```python
from build123d import *

# Parameters (mm, degrees)
SKETCH_1_R      = 2
SKETCH_1_R_2    = 9.5
EXTRUDE_2_DEPTH = 1.5


with BuildPart() as part:
    # 草图1 → 凸台-拉伸2 (new, symmetric)
    # profile 1 of 2: a face of its own
    with BuildSketch(Plane.XY):
        with BuildLine():
            Line((-30, 12.5), (-30, -22.5))
            Line((-30, -22.5), (30, -22.5))
            Line((30, -22.5), (30, 22.5))
            Line((30, 22.5), (-20, 22.5))
            Line((-20, 22.5), (-20, 14.5))
            ThreePointArc((-20, 14.5), (-18.585786438, 13.914213562), (-18, 12.5))
            ThreePointArc((-18, 12.5), (-20, 10.5), (-22, 12.5))
            Line((-22, 12.5), (-30, 12.5))
        make_face()
        with Locations((-20, -12.5)):
            Circle(SKETCH_1_R, mode=Mode.SUBTRACT)
        with Locations((20, -12.5)):
            Circle(SKETCH_1_R, mode=Mode.SUBTRACT)
        with Locations((0, 2.5)):
            Circle(SKETCH_1_R_2, mode=Mode.SUBTRACT)
        with Locations((20, 12.5)):
            Circle(SKETCH_1_R, mode=Mode.SUBTRACT)
    # profile 2 of 2: a face of its own
    with BuildSketch(Plane.XY):
        with BuildLine():
            Line((-30, 22.5), (-30, 12.5))
            Line((-30, 12.5), (-22, 12.5))
            ThreePointArc((-22, 12.5), (-21.414213562, 13.914213562), (-20, 14.5))
            Line((-20, 14.5), (-20, 22.5))
            Line((-20, 22.5), (-30, 22.5))
        make_face()
    extrude(amount=EXTRUDE_2_DEPTH, both=True)


solid = part.part
```
Geometry check sheet. Reference: the model listing, model coordinates, mm. Round coordinates to 2 decimals unless told otherwise and drop trailing zeros. Order: outer loops, then holes, each group sorted by start corner. A loop starts at its lowest first (then second) coordinate and runs counter-clockwise, first axis right, second up. Notation, with made-up numbers: (84, 14) - (114, 14) arc R13 cw to (114, 31) - close; hole circle Ø3 at (5, -30). An arc over 180 degrees is marked (long way). Use a Markdown table: item, result. Add a question column.
(1) Sectioned sample at C-C, the plane x = 20. Enter the section's corners in (y, z), and give its area (3 significant figures).
(2) Sectioned sample at B-B, the plane y = -12.5. Enter the section's corners in (x, z).
(3) Release check for a two-part mould opening along Y. For faces 1 (the cylindrical face through (19.74, 14.483, -0.021)), 2 (the flat face through (0, -22.5, 0)), 3 (the flat face through (-30, 0, 0)) record: pulls with the +Y half, pulls with the -Y half, needs draft (parallel to the pull), parting line crosses it, or undercut.
(4) Sectioned sample at A-A, the plane x = 0. Enter the section's corners in (y, z).
(5) Depth check by flat-ended pin: pin 1 (24.5 mm diameter, centred on x = 0, y = 2.5, fed in from +Z). Enter the tip coordinate at first touch or a pass-through.
(6) Sectioned sample at D-D, the plane y = 2.5. Enter the section's corners in (x, z), and give its area (3 significant figures).
(7) Material ranges on line 1 along Y through (x, z) = (-20, 0.75); line 2 along Y through (x, z) = (0, 0.05); line 3 along Y through (x, z) = (-4, 1.25), recorded low to high. Write a range as [from, to].
Answers below:
| question | item | result |
|---|---|---|
| 1 | outline | (-22.5, -1.5) - (-14.5, -1.5) - (-14.5, 1.5) - (-22.5, 1.5) - close; (-10.5, -1.5) - (10.5, -1.5) - (10.5, 1.5) - (-10.5, 1.5) - close; (14.5, -1.5) - (22.5, -1.5) - (22.5, 1.5) - (14.5, 1.5) - close |
| 1 | area | 111 mm² |
| 2 | outline | (-30, -1.5) - (-22, -1.5) - (-22, 1.5) - (-30, 1.5) - close; (-18, -1.5) - (18, -1.5) - (18, 1.5) - (-18, 1.5) - close; (22, -1.5) - (30, -1.5) - (30, 1.5) - (22, 1.5) - close |
| 3 | face 1 | undercut |
| 3 | face 2 | pulls with the -Y half |
| 3 | face 3 | needs draft |
| 4 | outline | (-22.5, -1.5) - (-7, -1.5) - (-7, 1.5) - (-22.5, 1.5) - close; (12, -1.5) - (22.5, -1.5) - (22.5, 1.5) - (12, 1.5) - close |
| 5 | pin 1 | z = 1.5 |
| 6 | outline | (-30, -1.5) - (-9.5, -1.5) - (-9.5, 1.5) - (-30, 1.5) - close; (9.5, -1.5) - (30, -1.5) - (30, 1.5) - (9.5, 1.5) - close |
| 6 | area | 123 mm² |
| 7 | line 1 | [-22.5, -14.5], [-10.5, 10.5], [14.5, 22.5] |
| 7 | line 2 | [-22.5, -7], [12, 22.5] |
| 7 | line 3 | [-22.5, -6.12], [11.12, 22.5] |
